For this review, use the dimensioned drawing (mm, ordinates from the lowest corner) and the shaded views. A direction names the side the tool comes from. Round coordinates to 2 decimals unless told otherwise and drop trailing zeros. Loops run counter-clockwise (first coordinate to the right, second up) from the corner with the lowest first, then second, coordinate; pieces in that order, holes last. Notation, with made-up numbers: (5, 0.25) - (18, 0.25) arc R11 ccw to (18, 10.25) - close; hole circle Ø4 at (39.5, 4). An arc over 180 degrees is marked (long way). Return JSON: item names as keys, results as strings. Group by question number.
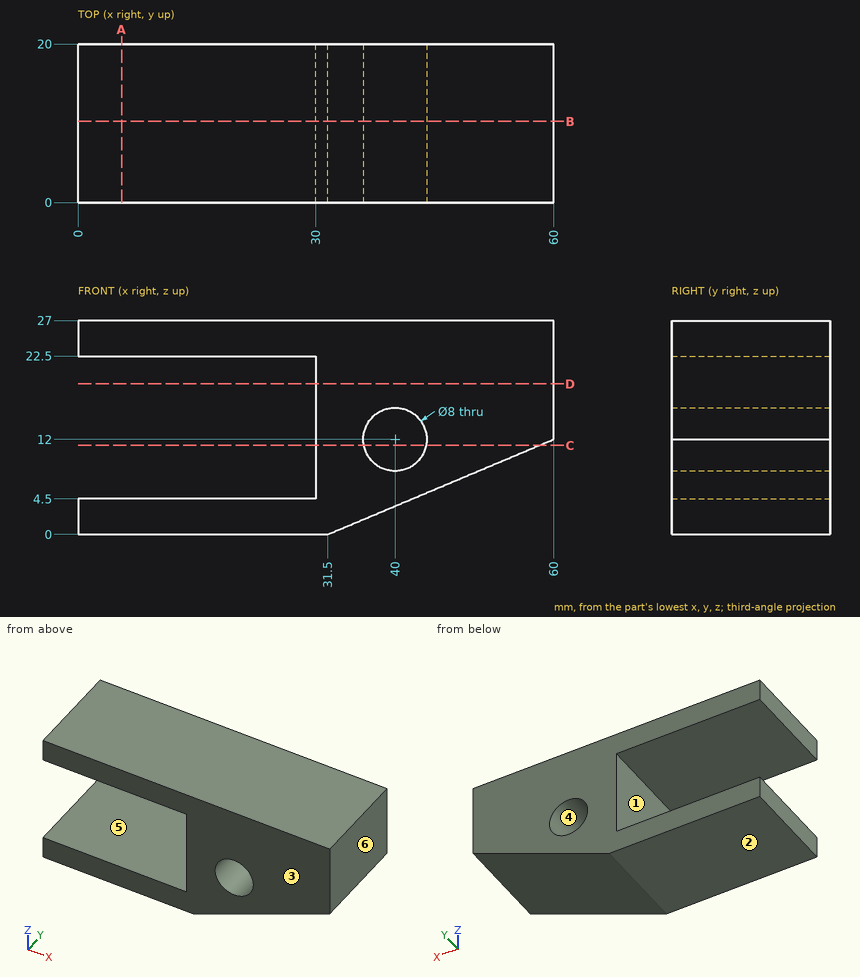
Q1. Add section A-A, the plane x = 5.5. State the section outline as (y, z) points, plus the area to 3 significant figures.
Q2. Tool access review of the marked faces 5 and 6: name each direction out of +Z, -Z, +X, -X, +Y, -Y from which nothing blocks a thin tool from reaching the whole face with its end or side.
Q3. Add section B-B, the plane y = 10.25. State the section outline as (x, z) points.
Q4. Add section C-C, the plane z = 11.25. State the section outline as (x, y) points, plus the area to 3 significant figures.
Q5. For line 1 (Z direction, x = 16, y = 14); line 2 (Z direction, x = 42.5, y = 3.25); line 3 (X direction, y = 19, z = 11.25), list the stretches that pass through material, from the lowest coordinate up.
Q6. Draft analysis for pull direction Z (two halves, no side actions). For the marked faces 1, 2, 3 and 4, state which applies: pulls with the +Z half, pulls with the -Z half, needs draft (parallel to the pull), parting line crosses it, or undercut.
Q7. Insertion check: pin 1 Ø6 at (x, z) = (12, 8.5) entering from +Y. The pin has a flat end and moves straight along its axis. Give the tip position at first contact, or say it passes through.
Q8. Add section D-D, the plane z = 19. State the section outline as (x, y) points.
Evaluation:
{
 "1": {"outline": "(0, 0) - (20, 0) - (20, 4.5) - (0, 4.5) - close; (0, 22.5) - (20, 22.5) - (20, 27) - (0, 27) - close", "area": "180 mm²"},
 "2": {"face 5": "-X, +Y, -Y", "face 6": "+Z, -Z, +X, +Y, -Y"},
 "3": {"outline": "(0, 0) - (31.5, 0) - (60, 12) - (60, 27) - (0, 27) - (0, 22.5) - (30, 22.5) - (30, 4.5) - (0, 4.5) - close; hole circle Ø8 at (40, 12)"},
 "4": {"outline": "(30, 0) - (36.07, 0) - (36.07, 20) - (30, 20) - close; (43.93, 0) - (58.22, 0) - (58.22, 20) - (43.93, 20) - close", "area": "407 mm²"},
 "5": {"line 1": "0 to 4.5, 22.5 to 27", "line 2": "4.63 to 8.88, 15.12 to 27", "line 3": "30 to 36.07, 43.93 to 58.22"},
 "6": {"face 1": "undercut", "face 2": "pulls with the -Z half", "face 3": "needs draft", "face 4": "undercut"},
 "7": {"pin 1": "through"},
 "8": {"outline": "(30, 0) - (60, 0) - (60, 20) - (30, 20) - close"}
}
